Input: part model. Units: mm. Frame: model coordinates. A direction names the side the tool comes from. Give positions to 0.01 mm unless a question says otherwise; leave off trailing zeros. Loops run counter-clockwise (first coordinate to the right, second up) from the corner with the lowest first, then second, coordinate; pieces in that order, holes last. Notation, with made-up numbers: (85.5, 74) -> (118.5, 74) arc R21 ccw to (118.5, 106) -> close; hole circle Ø1 at (76.5, 81). An arc over 180 degrees is marked (long way). Answer in a Markdown table with one row per item. Add a question column.
```python
from build123d import *


with BuildPart() as part:
    # Esquisse1 → Révolution1 (revolve)
    with BuildSketch(Plane(origin=(0, 0, 0), x_dir=(0, 0, -1), z_dir=(1, 0, 0)), mode=Mode.PRIVATE) as r_volution1_sk:
        Polygon((0, 0), (0, 40.25), (-18, 40.25), (-20, 42.25), (-20, 43), (1, 43), (3, 41), (3, 0), align=None)
    revolve(r_volution1_sk.sketch.rotate(Axis((0, 0, -3), (0, 0, 1)), 90), axis=Axis((0, 0, -3), (0, 0, 1)))  # turned: the seam where the file's is


solid = part.part
```
1) Reachability of faces 1 (the face through (-1, -1, 0)), 2 (the face through (1, -1, -3)) from +Z, -Z, +X, -X, +Y, -Y: full face, straight path, thin tool, end or side. Return the list, or none.
2) Pull-direction query (Y, two-part tool) for faces 3 (the face through (5.598, -42.634, 9.353)), 4 (the face through (-38.511, -12.128, 18.125)), 5 (the face through (32, 28, 20)); classes: +Y half, -Y half, draft (parallel to the pull), parting line (faces both ways), or undercut.
3) Section B-B on z = 3. Output: boundary loops of the cut face in (x, y), and give its area (3 significant figures).
4) Pin query (flat end, axial travel): pin 1 (1 mm diameter, centred on x = -3, y = 22, fed in from +Z); pin 2 (5 mm diameter, centred on y = 24, z = 2, fed in from +X); pin 3 (10 mm diameter, centred on y = 18, z = 2, fed in from +X). Return the tip coordinate at first contact, or that it passes through.
5) Section A-A on y = 0. Output: boundary loops of the cut face in (x, z), and give its area (3 significant figures).
6) Material intervals for line 1 along Y through (x, z) = (0, 5.25); line 2 along Z through (x, y) = (19, -0.5); line 3 along X through (y, z) = (-4.5, 7.5), sorted ascending.
Working result:
| question | item | result |
|---|---|---|
| 1 | face 1 | +Z |
| 1 | face 2 | -Z, +X, -X, +Y, -Y |
| 2 | face 3 | parting line |
| 2 | face 4 | undercut |
| 2 | face 5 | draft |
| 3 | outline | circle Ø86 at (0, 0); hole circle Ø80.5 at (0, 0) |
| 3 | area | 719 mm2 |
| 4 | pin 1 | stops at z = 0 |
| 4 | pin 2 | stops at x = 37.24 |
| 4 | pin 3 | stops at x = 40.99 |
| 5 | outline | (-43, -1) -> (-41, -3) -> (41, -3) -> (43, -1) -> (43, 20) -> (42.25, 20) -> (40.25, 18) -> (40.25, 0) -> (-40.25, 0) -> (-40.25, 18) -> (-42.25, 20) -> (-43, 20) -> close |
| 5 | area | 360 mm2 |
| 6 | line 1 | y = -43 to -40.25, 40.25 to 43 |
| 6 | line 2 | z = -3 to 0 |
| 6 | line 3 | x = -42.76 to -40, 40 to 42.76 |
